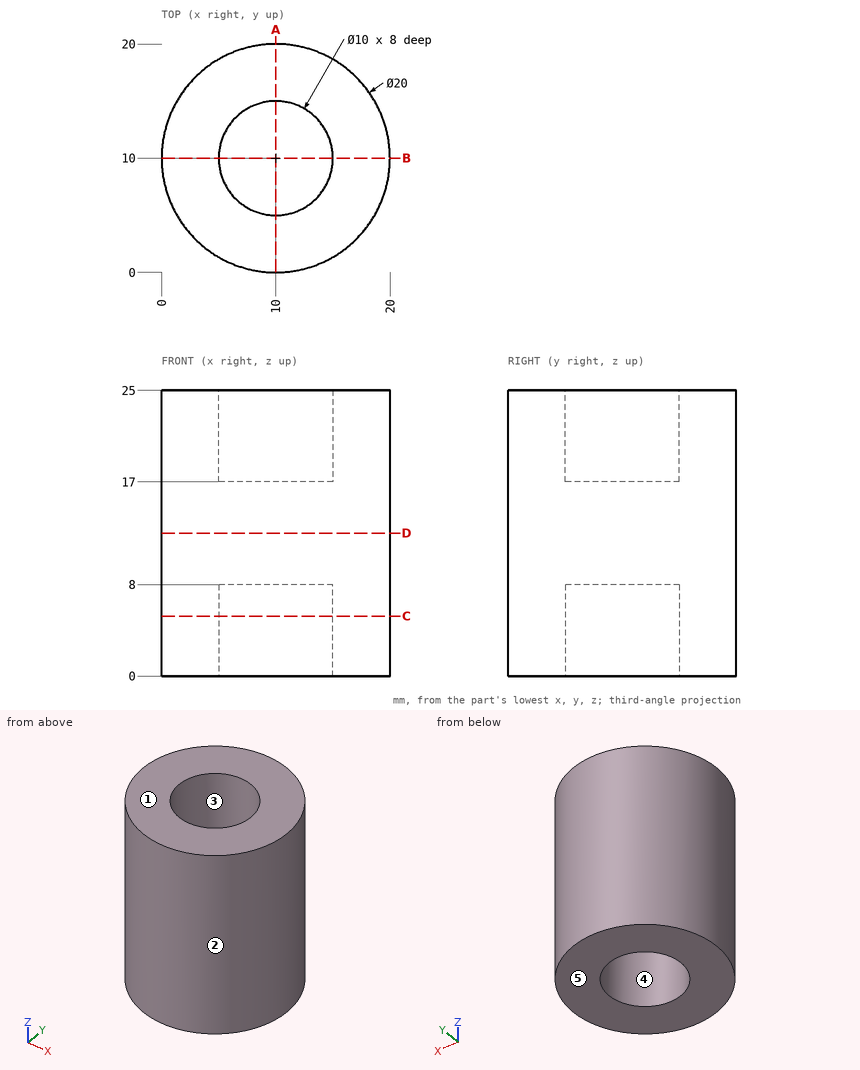
Drawing for the job (mm, zero at the part's lowest x, y, z). A direction names the side the tool comes from. Give positions to 0.01 mm unless a question says otherwise; leave off trailing zeros. Loops run counter-clockwise (first coordinate to the right, second up) from the corner with the lowest first, then second, coordinate; pieces in that order, holes last. Notation, with made-up numbers: M 34,-33.75 L 58,-33.75 A21 ccw 58,-11.75 Z; hole C -34.5,78.25 d4. An arc over 180 degrees is marked long. One line per question, with ' | ' between items. Start each with the question number.
1. Saw through at D-D on z = 12.5. Give the cut face in (x, y), plus the area to 3 significant figures.
2. Saw through at A-A on x = 10. Give the cut face in (y, z).
3. Two-plate mould, pull along Y, no slides. Class the marked faces 1, 2 and 3: pulls with the +Y half, pulls with the -Y half, needs draft (parallel to the pull), parting line crosses it, or undercut.
4. Saw through at C-C on z = 5.25. Give the cut face in (x, y), plus the area to 3 significant figures.
5. Flat gauge pins, fed straight in: pin 1 (3 mm diameter, centred on x = 7.5, z = 17, fed in from +Y); pin 2 (6 mm diameter, centred on x = 10, y = 10, fed in from -Z); pin 3 (6 mm diameter, centred on x = 10, y = 10, fed in from +Z); pin 4 (8 mm diameter, centred on x = 15, y = 12, fed in from -Z). Where does each tip first touch, or does it go through?
6. Probe L1, parallel to Y at x = 10, z = 3.75; L2, parallel to Y at x = 7, z = 23.5; L3, parallel to Z at x = 12, y = 14.25. List the from-to ranges inside material, lowest first. Write a range as from..to.
7. 3-axis set-ups, long thin cutter, end or side, ignore diameter. For the marked faces 4 and 5: which of +Z, -Z, +X, -X, +Y, -Y reach the whole face in a straight line?
Result sheet:
1) outline: C 10,10 d20 | area: 314 mm^2
2) outline: M 0,0 L 5,0 L 5,8 L 15,8 L 15,0 L 20,0 L 20,25 L 15,25 L 15,17 L 5,17 L 5,25 L 0,25 Z
3) face 1: needs draft | face 2: parting line crosses it | face 3: undercut
4) outline: C 10,10 d20; hole C 10,10 d10 | area: 236 mm^2
5) pin 1: stops at y = 19.95 | pin 2: stops at z = 8 | pin 3: stops at z = 17 | pin 4: stops at z = 0
6) L1: y = 0..5, 15..20 | L2: y = 0.46..6, 14..19.54 | L3: z = 8..17
7) face 4: -Z | face 5: -Z, +X, -X, +Y, -Y
